from build123d import *

# Parameters (mm, degrees)
F0_W     = 776
F0_H     = 100
F1_DEPTH = 12
F3_D     = 15
F5_D     = 5


with BuildPart() as f1:
    # F0 (on Front) → F1 (new body)
    with BuildSketch(Plane.XZ):
        with Locations((388, -50)):
            Rectangle(F0_W, F0_H)
    extrude(amount=-F1_DEPTH)

    # F3 (through all)
    with Locations(Plane.XZ):
        with Locations((100, -50), (676, -50)):
            Hole(F3_D / 2)

    # F5 (through all)
    with Locations(Plane.XZ):
        with Locations((300, -80), (476, -80)):
            Hole(F5_D / 2)


solid = f1.part
CAD build for the part. Positions are in the model's coordinates, mm. Round coordinates to 2 decimals unless told otherwise and drop trailing zeros. Loops run counter-clockwise (first coordinate to the right, second up) from the corner with the lowest first, then second, coordinate; pieces in that order, holes last.
(1) Two-plate mould, pull along Z, no slides. Class faces 1 (the cylindrical face through (101.63, 6.08, -57.32)), 2 (the flat face through (776, 6, -51)), 3 (the cylindrical face through (668.846, 6.084, -47.747)), 4 (the flat face through (383, 6, -100)): +Z half, -Z half, draft (parallel to the pull), parting line (faces both ways), or undercut.
(2) Cut at A-A (x = 676). Give the cut face in (y, z).
(3) Cut at B-B (z = -50). Give the cut face in (x, y).
(4) Wall check: line 1 along Z through (x, y) = (300, 9.25); line 2 along Z through (x, y) = (100, 7). Give the ranges that are in metal, low to high.
Findings below:
1. face 1: undercut
1. face 2: draft
1. face 3: undercut
1. face 4: -Z half
2. outline: (0, -100) - (12, -100) - (12, -57.5) - (0, -57.5) - close; (0, -42.5) - (12, -42.5) - (12, 0) - (0, 0) - close
3. outline: (0, 0) - (92.5, 0) - (92.5, 12) - (0, 12) - close; (107.5, 0) - (668.5, 0) - (668.5, 12) - (107.5, 12) - close; (683.5, 0) - (776, 0) - (776, 12) - (683.5, 12) - close
4. line 1: z = -100 to -82.5, -77.5 to 0
4. line 2: z = -100 to -57.5, -42.5 to 0
